Model file for the job. Use its own axes, mm. A direction names the side the tool comes from. Coordinates: 2 decimals unless noted, no trailing zeros. Order: outer loops, then holes, each group sorted by start corner. A loop starts at its lowest first (then second) coordinate and runs counter-clockwise, first axis right, second up. Notation, with made-up numbers: M 36,37.25 L 56,37.25 A20 cw 56,45.25 Z; hole C 69,1.5 d3. An arc over 180 degrees is marked long. Return JSON: item names as keys, results as strings.
```python
from build123d import *

# Parameters (mm, degrees)
BOSS_EXTRUDE1_DEPTH      = 325
BOSS_EXTRUDE1_DEPTH_BACK = 170
SKETCH2_R                = 2.95
SKETCH2_R_2              = 2.5
CUT_EXTRUDE1_DEPTH       = 2


with BuildPart() as part:
    # Sketch1 → Boss-Extrude1 (new, two sides: drawn at the far end of the back side and taken through both)
    with BuildSketch(Plane(origin=(0, 0, 0), x_dir=(0, 0, -1), z_dir=(1, 0, 0)).offset(-BOSS_EXTRUDE1_DEPTH_BACK)):
        Polygon((0, 20), (0, 0), (20, 0), (20, 2), (2, 2), (2, 20), align=None)
    extrude(amount=BOSS_EXTRUDE1_DEPTH + BOSS_EXTRUDE1_DEPTH_BACK)

    # Sketch2 → Cut-Extrude1 (cut)
    with BuildSketch(Plane(origin=(0, 2, 0), x_dir=(1, 0, 0), z_dir=(0, 1, 0))):
        with Locations(Location((0, 9.8, 0), (0, 0, 270))):
            Circle(SKETCH2_R)
        with Locations(Location((315, 11, 0), (0, 0, 270))):
            Circle(SKETCH2_R_2)
        with Locations(Location((-160, 11, 0), (0, 0, 270))):
            Circle(SKETCH2_R_2)
    extrude(amount=-CUT_EXTRUDE1_DEPTH, mode=Mode.SUBTRACT)


solid = part.part
```
Item 1: Drop flat-ended pins along their axis: pin 1 Ø5.5 at (x, y) = (34, 14) entering from -Z; pin 2 Ø1 at (x, z) = (128, -15.5) entering from -Y; pin 3 Ø9.5 at (x, z) = (0, -9.8) entering from +Y. Give the stop position or say it passes through.
Check result:
{"pin 1": "stops at z = -2", "pin 2": "stops at y = 0", "pin 3": "stops at y = 2"}
Item 2: Wall check: line 1 (X direction, y = 0.7, z = -9.8); line 2 (Y direction, x = 108.5, z = -7.75); line 3 (Z direction, x = -160, y = 1.55). Give the ranges that are in metal, low to high.
Check result:
{"line 1": "x = -170 to -162.19, -157.81 to -2.95, 2.95 to 312.81, 317.19 to 325", "line 2": "y = 0 to 2", "line 3": "z = -20 to -13.5, -8.5 to 0"}
Item 3: Saw through at B-B (z = -16.5). Write the cut outline in (x, y).
Check result:
{"outline": "M -170,0 L 325,0 L 325,2 L -170,2 Z"}
Item 4: 3-axis set-ups, long thin cutter, end or side, ignore diameter. For faces 1 (the flat face through (74, 0, -10)), 2 (the flat face through (74, 11, -2)): which of +Z, -Z, +X, -X, +Y, -Y reach the whole face in a straight line?
Check result:
{"face 1": "+Z, -Z, +X, -X, -Y", "face 2": "-Z, +X, -X, +Y"}
Item 5: Saw through at C-C (y = 8.75). Write the cut outline in (x, z).
Check result:
{"outline": "M -170,-2 L 325,-2 L 325,0 L -170,0 Z"}
Item 6: Saw through at A-A (x = 162.5). Write the cut outline in (y, z), and give its area (3 significant figures).
Check result:
{"outline": "M 0,-20 L 2,-20 L 2,-2 L 20,-2 L 20,0 L 0,0 Z", "area": "76.0 mm2"}
